```python
from build123d import *

# Parameters (mm, degrees)
BOSS_EXTRUDE1_DEPTH = 2.5
SKETCH3_W           = 2.5
SKETCH3_H           = 60
BOSS_EXTRUDE4_DEPTH = 2.5
BOSS_EXTRUDE5_DEPTH = 20
SKETCH7_R           = 3.75
BOSS_EXTRUDE6_DEPTH = 5.5
SKETCH9_R           = 3.75
BOSS_EXTRUDE7_DEPTH = 5.5
SKETCH10_R          = 1.05
CUT_EXTRUDE1_DEPTH  = 2.5
SKETCH12_R          = 1.05
CUT_EXTRUDE2_DEPTH  = 2.5
SKETCH14_W          = 5
SKETCH14_H          = 7.5
BOSS_EXTRUDE8_DEPTH = 10
SKETCH15_W          = 2.2
SKETCH15_H          = 12.5
SKETCH15_W_2        = 2.5
BOSS_EXTRUDE9_DEPTH = 10
SKETCH16_R          = 1.5
CUT_EXTRUDE3_DEPTH  = 114


with BuildPart() as part:
    # Sketch2 → Boss-Extrude1 (new body)
    with BuildSketch(Plane(origin=(0, 0, 0), x_dir=(1, 0, 0), z_dir=(0, 1, 0))):
        with BuildLine():
            Line((62.5, 25), (62.5, -25))
            ThreePointArc((62.5, -25), (53.127416998, -47.627416998), (30.5, -57))
            Line((30.5, -57), (23.5, -57))
            Line((23.5, -57), (23.5, -35))
            Line((23.5, -35), (30.5, -35))
            ThreePointArc((30.5, -35), (40.5, -25), (30.5, -15))
            Line((30.5, -15), (-38.5, -15))
            ThreePointArc((-38.5, -15), (-48.5, -25), (-38.5, -35))
            Line((-38.5, -35), (-31.5, -35))
            Line((-31.5, -35), (-31.5, -57))
            Line((-31.5, -57), (-38.5, -57))
            Line((-38.5, -57), (-62.5, -57))
            Line((-62.5, -57), (-62.5, 57))
            Line((-62.5, 57), (-38.5, 57))
            Line((-38.5, 57), (-31.5, 57))
            Line((-31.5, 57), (-31.5, 35))
            Line((-31.5, 35), (-38.5, 35))
            ThreePointArc((-38.5, 35), (-48.5, 25), (-38.5, 15))
            Line((-38.5, 15), (30.5, 15))
            ThreePointArc((30.5, 15), (40.5, 25), (30.5, 35))
            Line((30.5, 35), (23.5, 35))
            Line((23.5, 35), (23.5, 57))
            Line((23.5, 57), (30.5, 57))
            ThreePointArc((30.5, 57), (53.127416998, 47.627416998), (62.5, 25))
        make_face()
    extrude(amount=BOSS_EXTRUDE1_DEPTH)

    # Sketch3 → Boss-Extrude4 (add)
    # profile 1 of 3: a face of its own
    with BuildSketch(Plane(origin=(0, 2.5, 0), x_dir=(1, 0, 0), z_dir=(0, 1, 0))):
        with BuildLine():
            Line((30.5, -40.000579699), (30.5, -35))
            Line((30.5, -35), (23.5, -35))
            Line((23.5, -35), (23.5, -57))
            Line((23.5, -57), (30.5, -57))
            Line((30.5, -57), (30.5, -47.5))
            ThreePointArc((30.5, -47.5), (53, -25), (30.5, -2.5))
            Line((30.5, -2.5), (-38.5, -2.5))
            ThreePointArc((-38.5, -2.5), (-61, -25), (-38.5, -47.5))
            Line((-38.5, -47.5), (-38.5, -57))
            Line((-38.5, -57), (-31.5, -57))
            Line((-31.5, -57), (-31.5, -35))
            Line((-31.5, -35), (-38.5, -35))
            Line((-38.5, -35), (-38.5, -40.000579699))
            ThreePointArc((-38.5, -40.000579699), (-53.500434773, -25.065938667), (-38.631876061, -10))
            Line((-38.631876061, -10), (30.368123939, -10))
            ThreePointArc((30.368123939, -10), (45.500434773, -24.934061333), (30.5, -40.000579699))
        make_face()
        with BuildLine():
            Line((30.368123939, -7.5), (-38.631876061, -7.5))
            ThreePointArc((-38.631876061, -7.5), (-56.000372665, -25.065938498), (-38.5, -42.500496887))
            Line((-38.5, -42.500496887), (-38.5, -45))
            ThreePointArc((-38.5, -45), (-58.5, -25), (-38.5, -5))
            Line((-38.5, -5), (30.5, -5))
            ThreePointArc((30.5, -5), (50.5, -25), (30.5, -45))
            Line((30.5, -45), (30.5, -42.500496887))
            ThreePointArc((30.5, -42.500496887), (48.000372665, -24.934061502), (30.368123939, -7.5))
        make_face(mode=Mode.SUBTRACT)
    # profile 2 of 3: a face of its own
    with BuildSketch(Plane(origin=(0, 2.5, 0), x_dir=(1, 0, 0), z_dir=(0, 1, 0))):
        with BuildLine():
            Line((30.5, 57), (30.5, 47.5))
            ThreePointArc((30.5, 47.5), (53, 25), (30.5, 2.5))
            Line((30.5, 2.5), (-38.5, 2.5))
            ThreePointArc((-38.5, 2.5), (-61, 25), (-38.5, 47.5))
            Line((-38.5, 47.5), (-38.5, 57))
            Line((-38.5, 57), (-31.5, 57))
            Line((-31.5, 57), (-31.5, 35))
            Line((-31.5, 35), (-38.5, 35))
            Line((-38.5, 35), (-38.5, 40.000579699))
            ThreePointArc((-38.5, 40.000579699), (-53.500434773, 25.065938667), (-38.631876061, 10))
            Line((-38.631876061, 10), (30.368123939, 10))
            ThreePointArc((30.368123939, 10), (45.500434773, 24.934061333), (30.5, 40.000579699))
            Line((30.5, 40.000579699), (30.5, 35))
            Line((30.5, 35), (23.5, 35))
            Line((23.5, 35), (23.5, 57))
            Line((23.5, 57), (30.5, 57))
        make_face()
        with BuildLine():
            Line((30.5, 42.500496887), (30.5, 45))
            ThreePointArc((30.5, 45), (50.5, 25), (30.5, 5))
            Line((30.5, 5), (-38.5, 5))
            ThreePointArc((-38.5, 5), (-58.5, 25), (-38.5, 45))
            Line((-38.5, 45), (-38.5, 42.500496887))
            ThreePointArc((-38.5, 42.500496887), (-56.000372665, 25.065938498), (-38.631876061, 7.5))
            Line((-38.631876061, 7.5), (30.368123939, 7.5))
            ThreePointArc((30.368123939, 7.5), (48.000372665, 24.934061502), (30.5, 42.500496887))
        make_face(mode=Mode.SUBTRACT)
    # profile 3 of 3: a face of its own
    with BuildSketch(Plane(origin=(0, 2.5, 0), x_dir=(1, 0, 0), z_dir=(0, 1, 0))):
        with Locations((56.25, 0)):
            Rectangle(SKETCH3_W, SKETCH3_H)
    extrude(amount=BOSS_EXTRUDE4_DEPTH)

    # Sketch6 → Boss-Extrude5 (add)
    with BuildSketch(Plane(origin=(0, 5, 0), x_dir=(1, 0, 0), z_dir=(0, 1, 0))):
        Polygon((-38.5, -35), (-31.5, -35), (-31.5, -57), (-38.5, -57), (-38.5, -54.5), (-34, -54.5), (-34, -37.5), (-38.5, -37.5), align=None)
        Polygon((30.5, -35), (23.5, -35), (23.5, -57), (30.5, -57), (30.5, -54.5), (26, -54.5), (26, -37.5), (30.5, -37.5), align=None)
        Polygon((30.5, 37.5), (30.5, 35), (23.5, 35), (23.5, 57), (30.5, 57), (30.5, 54.5), (26, 54.5), (26, 37.5), align=None)
        Polygon((-38.5, 37.5), (-38.5, 35), (-31.5, 35), (-31.5, 57), (-38.5, 57), (-38.5, 54.5), (-34, 54.5), (-34, 37.5), align=None)
    extrude(amount=BOSS_EXTRUDE5_DEPTH)

    # Sketch7 → Boss-Extrude6 (add)
    with BuildSketch(Plane.ZY.offset(-23.5)):
        with Locations(Location((46, 13.75, 0), (0, 0, 180))):
            Circle(SKETCH7_R)
    extrude(amount=BOSS_EXTRUDE6_DEPTH)

    # Sketch9 → Boss-Extrude7 (add)
    with BuildSketch(Plane.ZY.offset(-23.5)):
        with Locations(Location((-46, 13.75, 0), (0, 0, 180))):
            Circle(SKETCH9_R)
    extrude(amount=BOSS_EXTRUDE7_DEPTH)

    # Sketch10 → Cut-Extrude1 (cut)
    with BuildSketch(Plane(origin=(-31.5, 0, 0), x_dir=(0, 0, -1), z_dir=(1, 0, 0))):
        with Locations((-42.5, 22)):
            Circle(SKETCH10_R)
        with Locations(Location((-49.5, 22, 0), (0, 0, 180))):
            Circle(SKETCH10_R)
        with Locations((-49.5, 8)):
            Circle(SKETCH10_R)
        with Locations(Location((-42.5, 8, 0), (0, 0, 180))):
            Circle(SKETCH10_R)
    extrude(amount=-CUT_EXTRUDE1_DEPTH, mode=Mode.SUBTRACT)

    # Sketch12 → Cut-Extrude2 (cut)
    with BuildSketch(Plane(origin=(-31.5, 0, 0), x_dir=(0, 0, -1), z_dir=(1, 0, 0))):
        with Locations((49.5, 22)):
            Circle(SKETCH12_R)
        with Locations(Location((42.5, 22, 0), (0, 0, 180))):
            Circle(SKETCH12_R)
        with Locations((42.5, 8)):
            Circle(SKETCH12_R)
        with Locations(Location((49.5, 8, 0), (0, 0, 180))):
            Circle(SKETCH12_R)
    extrude(amount=-CUT_EXTRUDE2_DEPTH, mode=Mode.SUBTRACT)

    # Sketch14 → Boss-Extrude8 (add)
    with BuildSketch(Plane(origin=(0, 2.5, 0), x_dir=(1, 0, 0), z_dir=(0, 1, 0))):
        with Locations((-60, 0)):
            Rectangle(SKETCH14_W, SKETCH14_H)
        with Locations((-60, -53.25)):
            Rectangle(SKETCH14_W, SKETCH14_H)
        with Locations((-60, 53.25)):
            Rectangle(SKETCH14_W, SKETCH14_H)
    extrude(amount=BOSS_EXTRUDE8_DEPTH)

    # Sketch15 → Boss-Extrude9 (add)
    with BuildSketch(Plane.ZY.offset(62.5)):
        with Locations((0, 6.25)):
            Rectangle(SKETCH15_W, SKETCH15_H)
        with Locations((55.75, 6.25)):
            Rectangle(SKETCH15_W_2, SKETCH15_H)
        with Locations((50.75, 6.25)):
            Rectangle(SKETCH15_W_2, SKETCH15_H)
        with Locations((-50.75, 6.25)):
            Rectangle(SKETCH15_W_2, SKETCH15_H)
        with Locations((-55.75, 6.25)):
            Rectangle(SKETCH15_W_2, SKETCH15_H)
    extrude(amount=BOSS_EXTRUDE9_DEPTH)

    # Sketch16 → Cut-Extrude3 (cut)
    with BuildSketch(Plane.XY.offset(57)):
        with Locations((-68.75, 9.375)):
            Circle(SKETCH16_R)
        with Locations((-68.75, 3.125)):
            Circle(SKETCH16_R)
    extrude(amount=-CUT_EXTRUDE3_DEPTH, mode=Mode.SUBTRACT)


solid = part.part
```
Part model, mm, in its own coordinate system. A direction names the side the tool comes from. Round coordinates to 2 decimals unless told otherwise and drop trailing zeros. Use one line per item in the form item = value. Start each with the question number.
Item 1: Tool access for faces 4 (the flat face through (-57.5, 7, -53)), 5 (the cylindrical face through (40.5, 1.2, -24.8)), 6 (the cylindrical face through (48, 4, -25)): list every direction of +Z, -Z, +X, -X, +Y, -Y with a clear straight run to the whole face (end or side of a thin tool).
Item 2: Band-saw the part on A-A (y = 19.25). Give the number of separate pieces and of enclosed holes in the cut face, plus the area to 3 significant figures.
Item 3: Two-plate mould, pull along X, no slides. Class faces 1 (the cylindrical face through (53, 4, 25)), 2 (the cylindrical face through (53.37, 1.23, 47.38)), 3 (the flat face through (-67, 6, -54.5)): released by +X, released by -X, zero draft, split by the parting line, or undercut.
Item 4: Drop flat-ended pins along their axis: pin 1 Ø8 at (y, z) = (20, 41) entering from +X; pin 2 Ø0.8 at (x, y) = (-3.5, 4) entering from -Z; pin 3 Ø4 at (y, z) = (9.5, -0.5) entering from +X; pin 4 Ø1.8 at (x, y) = (-68.75, 3.125) entering from +Z. Give the stop position or say it passes through.
Item 5: Drill centre lines: line 1 along Y through (x, z) = (-32.8, -49.5); line 2 along Z through (x, y) = (-67, 11); line 3 along Y through (x, z) = (-32, 42). Where is each one in solid material? Low to high.
Data:
q1.face_4 = -Z, +Y
q1.face_5 = +Y, -Y
q1.face_6 = +Y
q2.separate_pieces = 4
q2.enclosed_holes = 0
q2.area = 310 mm^2
q3.face_1 = undercut
q3.face_2 = released by +X
q3.face_3 = zero draft
q4.pin_1 = 30.5
q4.pin_2 = -10
q4.pin_3 = -57.5
q4.pin_4 = through
q5.line_1 = 0 to 6.95, 9.05 to 20.95, 23.05 to 25
q5.line_2 = -57 to -54.5, -52 to -49.5, -1.1 to 1.1, 49.5 to 52, 54.5 to 57
q5.line_3 = 0 to 7.08, 8.92 to 21.08, 22.92 to 25
